Can you work these out from the model? Positions are in its coordinate system, mm. Face numbers are marked on the shaded views. A direction names the side the tool comes from. Coordinates: 2 decimals unless noted, no trailing zeros. Loops run counter-clockwise (first coordinate to the right, second up) from the corner with the lowest first, then second, coordinate; pieces in that order, holes last. Notation, with made-up numbers: (48, -1.5) -> (103, -1.5) arc R10 cw to (103, 2.5) -> close; hole circle Ø1 at (70.5, -14.75). An arc over 180 degrees is marked (long way). Use one line per item in the form item = value. Start each with the question number.
(1) Imagine slicing it at C-C (z = 26). List the corners of the cut face in (x, y) for me, plus the area to 3 significant figures.
(2) I'm going to push flat-ended pins straight in: pin 1 (3 mm diameter, centred on x = 92.5, y = 18.5, fed in from +Z); pin 2 (1.5 mm diameter, centred on y = 62, z = 36.5, fed in from -X). Where does each tip first touch, or does it pass through?
(3) On a 3-axis mill with a long thin cutter (end or side, diameter ignored), from which of +Z, -Z, +X, -X, +Y, -Y can I reach the whole of each face in a straight line? I mean the marked faces 4 and 5. Say none if no direction works.
(4) Thinking about a two-plate mould opening in X: for the marked faces 1, 2 and 3, which applies, released by +X, released by -X, zero draft, split by the parting line, or undercut?
(5) Imagine slicing it at A-A (x = 60). List the corners of the cut face in (y, z) for me.
(6) I need wall thicknesses on line 1 (Y direction, x = 60, z = 29); line 2 (Y direction, x = 60, z = 41); line 3 (Z direction, x = 18.5, y = 60). Which ranges of each line are inside material? Lowest first, please. Write a range as [from, to].
(7) Imagine slicing it at D-D (x = 88.5). List the corners of the cut face in (y, z) for me.
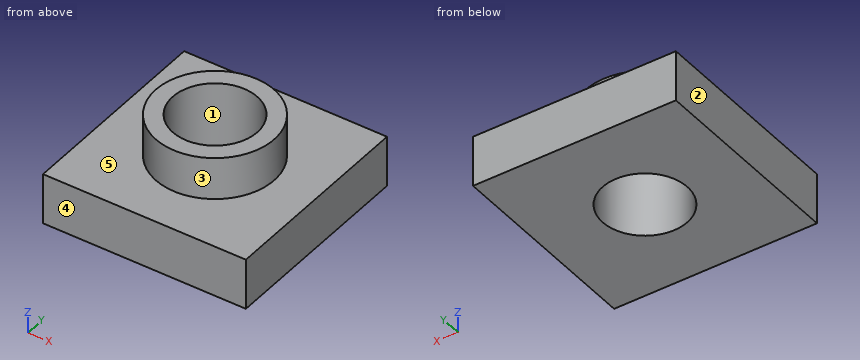
```python
from build123d import *

# Parameters (mm, degrees)
SKETCH_1_W      = 120
SKETCH_1_H      = 120
SKETCH_1_R      = 25
EXTRUDE_1_DEPTH = 30
SKETCH_2_R      = 35
SKETCH_2_R_2    = 25
EXTRUDE_2_DEPTH = 25


with BuildPart() as part:
    # 草圖1 → 填料-伸長1 (new body)
    with BuildSketch(Plane.XY):
        with Locations((60, 60)):
            Rectangle(SKETCH_1_W, SKETCH_1_H)
        with Locations((60, 60)):
            Circle(SKETCH_1_R, mode=Mode.SUBTRACT)
    extrude(amount=EXTRUDE_1_DEPTH)

    # 草圖2 → 填料-伸長2 (add)
    with BuildSketch(Plane.XY.offset(30)):
        with Locations(Location((60, 60, 0), (0, 0, 180))):
            Circle(SKETCH_2_R)
        with Locations((60, 60)):
            Circle(SKETCH_2_R_2, mode=Mode.SUBTRACT)
    extrude(amount=EXTRUDE_2_DEPTH)


solid = part.part
```
Worked out:
q1.outline = (0, 0) -> (120, 0) -> (120, 120) -> (0, 120) -> close; hole circle Ø50 at (60, 60)
q1.area = 12,400 mm2
q2.pin_1 = 30
q2.pin_2 = 25.02
q3.face_4 = +Z, -Z, +X, -X, -Y
q3.face_5 = +Z
q4.face_1 = undercut
q4.face_2 = released by -X
q4.face_3 = split by the parting line
q5.outline = (0, 0) -> (35, 0) -> (35, 55) -> (25, 55) -> (25, 30) -> (0, 30) -> close; (85, 0) -> (120, 0) -> (120, 30) -> (95, 30) -> (95, 55) -> (85, 55) -> close
q6.line_1 = [0, 35], [85, 120]
q6.line_2 = [25, 35], [85, 95]
q6.line_3 = [0, 30]
q7.outline = (0, 0) -> (120, 0) -> (120, 30) -> (80.32, 30) -> (80.32, 55) -> (39.68, 55) -> (39.68, 30) -> (0, 30) -> close
